Design review of the part built by this model. Coordinates are the model's own, in mm. A direction names the side the tool comes from. Give positions to 0.01 mm unless a question says otherwise; leave off trailing zeros. Loops run counter-clockwise (first coordinate to the right, second up) from the corner with the lowest first, then second, coordinate; pieces in that order, holes last.
from build123d import *

# Parameters (mm, degrees)
F1_DEPTH = 63.5
F0_W     = 25.4
F0_H     = 19.05
F2_DEPTH = 25.4
F4_DEPTH = 19.05
F5_R     = 6.35
F6_R     = 8.4119474029
F7_DEPTH = 19.051


with BuildPart() as f1:
    # F0 (on Front) → F1 (new body, symmetric)
    with BuildSketch(Plane.XZ):
        Polygon((-41.275, -9.525), (41.275, -9.525), (41.275, 9.525), (22.225, 9.525), (-41.275, 9.525), align=None)
    extrude(amount=F1_DEPTH, both=True)

    # F0 (on Front) → F2 (join, symmetric)
    with BuildSketch(Plane.XZ):
        with BuildLine():
            Line((22.225, 9.525), (41.275, 9.525))
            Line((41.275, 9.525), (41.275, 27.0002))
            ThreePointArc((41.275, 27.0002), (45.9246798487, 38.2255201513), (57.15, 42.8752))
            Line((57.15, 42.8752), (60.325, 42.8752))
            Line((60.325, 42.8752), (60.325, 61.9252))
            Line((60.325, 61.9252), (57.15, 61.9252))
            add(Edge.make_bspline(
                [(52.4539686953, 61.608044703), (54.0535682544, 61.7343536361), (55.620779482, 61.8398573918), (57.15, 61.9252)],
                knots=[106.9681475328, 106.9681475328, 106.9681475328, 106.9681475328, 111.5045361635, 111.5045361635, 111.5045361635, 111.5045361635], degree=3))
            ThreePointArc((52.4539686953, 61.608044703), (30.8463451369, 49.9756948987), (22.225, 27.0002))
            Line((22.225, 27.0002), (22.225, 9.525))
        make_face()
        with Locations((73.025, 52.4002)):
            Rectangle(F0_W, F0_H)
    extrude(amount=F2_DEPTH, both=True)

    # F0 (on Front) → F3 (revolve)
    with BuildSketch(Plane.XZ):
        Polygon((85.725, 61.9252), (85.725, 42.8752), (85.725, 34.925), (111.125, 34.925), (111.125, 66.675), (85.725, 66.675), align=None)
    revolve(axis=Axis((85.725, 0, 50.8), (0, 0, 1)))

    # F0 (on Front) → F4 (join, symmetric)
    with BuildSketch(Plane.XZ):
        with BuildLine():
            add(Edge.make_bspline(
                [(-41.275, 9.525), (-40.9916978958, 44.0832673995), (14.7353745544, 58.6296771756), (52.4539686953, 61.608044703)],
                knots=[0, 0, 0, 0, 106.9681475328, 106.9681475328, 106.9681475328, 106.9681475328], degree=3))
            Line((-41.275, 9.525), (22.225, 9.525))
            Line((22.225, 9.525), (22.225, 27.0002))
            ThreePointArc((22.225, 27.0002), (30.8463451369, 49.9756948987), (52.4539686953, 61.608044703))
        make_face()
    extrude(amount=F4_DEPTH, both=True)

    # F5
    f5_edges = [f1.edges().sort_by_distance(p)[0] for p in [
        (41.275, -63.5, 0),
        (-41.275, -63.5, 0),
        (41.275, 63.5, 0),
        (-41.275, 63.5, 0),
    ]]
    fillet(f5_edges, radius=F5_R)

    # F6 (on face) → F7 (cut, through all)
    with BuildSketch(Plane.XY.offset(9.525)):
        with Locations((-21.275, -43.5)):
            Circle(F6_R)
    extrude(amount=-F7_DEPTH, mode=Mode.SUBTRACT)


solid = f1.part
Q1. Take a section at D-D (x = 95). Give the boundary of the cut face in (y, z) (3 decimals).
Results:
outline: (-23.646, 34.925) - (23.646, 34.925) - (23.646, 66.675) - (-23.646, 66.675) - close
Q2. Insertion check: pin 1 (14.5 mm diameter, centred on x = 72.5, y = 0.5, fed in from -Z) (3 decimals); pin 2 (3 mm diameter, centred on x = 24, z = 23.5, fed in from -Y); pin 3 (12 mm diameter, centred on x = -3, y = -2.5, fed in from +Z). Each pin has a flat end and moves straight along its axis. Give the tip position at first contact, or say it passes through.
Results:
pin 1: stops at z = 34.925
pin 2: stops at y = -25.4
pin 3: stops at z = 51.86
Q3. Take a section at C-C (y = 35.5). Give the boundary of the cut face in (x, z) (3 decimals).
Results:
outline: (-41.275, -9.525) - (41.275, -9.525) - (41.275, 9.525) - (-41.275, 9.525) - close
Q4. Tool access review of faces 1 (the face through (60, -2, 61.925)), 2 (the face through (22.225, -22, 18)), 3 (the face through (60, 2, 42.875)): name each direction out of +Z, -Z, +X, -X, +Y, -Y from which nothing blocks a thin tool from reaching the whole face with its end or side.
Results:
face 1: +Z, -X
face 2: +Z, -X, -Y
face 3: -Z
Q5. Wall thickness on line 1 (X direction, y = -43, z = -4) (3 decimals); line 2 (Y direction, x = 10, z = 36); line 3 (Y direction, x = 37, z = 48.5): over which ranges is each line inside the solid? List them lowest first.
Results:
line 1: x = -41.275 to -29.672, -12.878 to 41.275
line 2: y = -19.05 to 19.05
line 3: y = -25.4 to 25.4
Q6. Take a section at B-B (x = 76). Give the boundary of the cut face in (y, z) (3 decimals).
Results:
outline: (-25.4, 42.875) - (-23.465, 42.875) - (-23.465, 34.925) - (23.465, 34.925) - (23.465, 42.875) - (25.4, 42.875) - (25.4, 61.925) - (23.465, 61.925) - (23.465, 66.675) - (-23.465, 66.675) - (-23.465, 61.925) - (-25.4, 61.925) - close
Q7. Take a section at A-A (y = -43.5). Give the boundary of the cut face in (x, z) (3 decimals).
Results:
outline: (-41.275, -9.525) - (-29.687, -9.525) - (-29.687, 9.525) - (-41.275, 9.525) - close; (-12.863, -9.525) - (41.275, -9.525) - (41.275, 9.525) - (-12.863, 9.525) - close
Q8. Draft analysis for pull direction X (two halves, no side actions). For faces 4 (the face through (46, -25.4, 42)), 5 (the face through (45.8, -0.4, 38.1)), 6 (the face through (31.08, 22.18, 50.24)), 7 (the face through (39.365, -61.689, 0.133)), state which applies: pulls with the +X half, pulls with the -X half, needs draft (parallel to the pull), parting line crosses it, or undercut.
Results:
face 4: needs draft
face 5: undercut
face 6: pulls with the -X half
face 7: pulls with the +X half
